```python
from build123d import *

# Parameters (mm, degrees)
SKETCH_1_R        = 1
EXTRUDE_1_DEPTH   = 1
SKETCH_1_2_R      = 1
EXTRUDE_1_2_DEPTH = 8
SKETCH_1_3_R      = 1
EXTRUDE_2_DEPTH   = 10
SCALE_4_SCALE     = 1.5


with BuildPart() as part:
    # 草图1 → Extrude 1 (new body)
    with BuildSketch(Plane.XY):
        with BuildLine():
            Line((-23.446136356, -44.161959762), (-25.73775467, -42.866863479))
            Line((-25.73775467, -42.866863479), (-26.834295942, -39.938466016))
            ThreePointArc((-26.834295942, -39.938466016), (-28.201527977, -38.125336415), (-30.335428898, -37.348658075))
            Line((-30.335428898, -37.348658075), (-33.334907776, -37.164700371))
            Line((-33.334907776, -37.164700371), (-33.842709051, -34.202800331))
            ThreePointArc((-33.842709051, -34.202800331), (-34.84597704, -32.165592505), (-36.7965457, -31.002818113))
            Line((-36.7965457, -31.002818113), (-39.708425324, -30.260072511))
            Line((-39.708425324, -30.260072511), (-39.652227319, -27.255483394))
            ThreePointArc((-39.652227319, -27.255483394), (-40.255989993, -25.066366444), (-41.954126526, -23.558687864))
            Line((-41.954126526, -23.558687864), (-44.675252109, -22.283466496))
            Line((-44.675252109, -22.283466496), (-44.057045667, -19.342627369))
            ThreePointArc((-44.057045667, -19.342627369), (-44.239914432, -17.079151855), (-45.625461503, -15.279979352))
            Line((-45.625461503, -15.279979352), (-48.059435816, -13.517457571))
            Line((-48.059435816, -13.517457571), (-46.901121207, -10.744549126))
            ThreePointArc((-46.901121207, -10.744549126), (-46.656617846, -8.486899797), (-47.680491761, -6.459969953))
            Line((-47.680491761, -6.459969953), (-49.741090048, -4.272585973))
            Line((-49.741090048, -4.272585973), (-48.083701146, -1.765839874))
            ThreePointArc((-48.083701146, -1.765839874), (-47.420487313, 0.406004917), (-48.046416828, 2.588887101))
            Line((-48.046416828, 2.588887101), (-49.660641368, 5.123644113))
            Line((-49.660641368, 5.123644113), (-47.562892001, 7.275425136))
            ThreePointArc((-47.562892001, 7.275425136), (-46.504462376, 9.284526705), (-46.710273625, 11.546031539))
            Line((-46.710273625, 11.546031539), (-47.82093971, 14.338366552))
            Line((-47.82093971, 14.338366552), (-45.357143694, 16.058954583))
            ThreePointArc((-45.357143694, 16.058954583), (-43.940993675, 17.834139505), (-43.719395692, 20.094152054))
            Line((-43.719395692, 20.094152054), (-44.287157421, 23.045145208))
            Line((-44.287157421, 23.045145208), (-41.54459596, 24.273587558))
            ThreePointArc((-41.54459596, 24.273587558), (-39.820893366, 25.751969023), (-39.17973637, 27.930427214))
            Line((-39.17973637, 27.930427214), (-39.184480502, 30.935538106))
            Line((-39.184480502, 30.935538106), (-36.260310201, 31.628316593))
            ThreePointArc((-36.260310201, 31.628316593), (-34.290118058, 32.757522199), (-33.252115355, 34.777253066))
            Line((-33.252115355, 34.777253066), (-32.693673826, 37.730024144))
            Line((-32.693673826, 37.730024144), (-29.691484877, 37.862596744))
            ThreePointArc((-29.691484877, 37.862596744), (-27.544598222, 38.602623821), (-26.146521576, 40.39207739))
            Line((-26.146521576, 40.39207739), (-25, 43.301270189))
            ThreePointArc((-25, 43.301270189), (-24.226890609, 43.73851588), (-23.446136356, 44.161959762))
            ThreePointArc((-23.446136356, 44.161959762), (-21.212806241, 47.755648425), (-21.906244367, 51.929556087))
            ThreePointArc((-21.906244367, 51.929556087), (-24.232021318, 53.76021953), (-27.179564099, 53.490852446))
            ThreePointArc((-27.179564099, 53.490852446), (-59.999999835, 0.004450967), (-27.1875, -53.486819346))
            Line((-27.1875, -53.486819346), (-27.179564099, -53.490852446))
            ThreePointArc((-27.179564099, -53.490852446), (-24.232021318, -53.76021953), (-21.906244367, -51.929556087))
            ThreePointArc((-21.906244367, -51.929556087), (-21.212806241, -47.755648425), (-23.446136356, -44.161959762))
        make_face()
        with Locations((-31.620079453, -45.001895242)):
            Circle(SKETCH_1_R, mode=Mode.SUBTRACT)
        with Locations((-55, 0)):
            Circle(SKETCH_1_R, mode=Mode.SUBTRACT)
        with Locations((-28.000624989, 47.338831842)):
            Circle(SKETCH_1_R, mode=Mode.SUBTRACT)
    extrude(amount=EXTRUDE_1_DEPTH)

    # 草图1<2> → Extrude 1 2 (add)
    with BuildSketch(Plane.XY):
        with BuildLine():
            Line((-23.446136356, -44.161959762), (-25.73775467, -42.866863479))
            Line((-25.73775467, -42.866863479), (-26.834295942, -39.938466016))
            ThreePointArc((-26.834295942, -39.938466016), (-28.201527977, -38.125336415), (-30.335428898, -37.348658075))
            Line((-30.335428898, -37.348658075), (-33.334907776, -37.164700371))
            Line((-33.334907776, -37.164700371), (-33.842709051, -34.202800331))
            ThreePointArc((-33.842709051, -34.202800331), (-34.84597704, -32.165592505), (-36.7965457, -31.002818113))
            Line((-36.7965457, -31.002818113), (-39.708425324, -30.260072511))
            Line((-39.708425324, -30.260072511), (-39.652227319, -27.255483394))
            ThreePointArc((-39.652227319, -27.255483394), (-40.255989993, -25.066366444), (-41.954126526, -23.558687864))
            Line((-41.954126526, -23.558687864), (-44.675252109, -22.283466496))
            Line((-44.675252109, -22.283466496), (-44.057045667, -19.342627369))
            ThreePointArc((-44.057045667, -19.342627369), (-44.239914432, -17.079151855), (-45.625461503, -15.279979352))
            Line((-45.625461503, -15.279979352), (-48.059435816, -13.517457571))
            Line((-48.059435816, -13.517457571), (-46.901121207, -10.744549126))
            ThreePointArc((-46.901121207, -10.744549126), (-46.656617846, -8.486899797), (-47.680491761, -6.459969953))
            Line((-47.680491761, -6.459969953), (-49.741090048, -4.272585973))
            Line((-49.741090048, -4.272585973), (-48.083701146, -1.765839874))
            ThreePointArc((-48.083701146, -1.765839874), (-47.420487313, 0.406004917), (-48.046416828, 2.588887101))
            Line((-48.046416828, 2.588887101), (-49.660641368, 5.123644113))
            Line((-49.660641368, 5.123644113), (-47.562892001, 7.275425136))
            ThreePointArc((-47.562892001, 7.275425136), (-46.504462376, 9.284526705), (-46.710273625, 11.546031539))
            Line((-46.710273625, 11.546031539), (-47.82093971, 14.338366552))
            Line((-47.82093971, 14.338366552), (-45.357143694, 16.058954583))
            ThreePointArc((-45.357143694, 16.058954583), (-43.940993675, 17.834139505), (-43.719395692, 20.094152054))
            Line((-43.719395692, 20.094152054), (-44.287157421, 23.045145208))
            Line((-44.287157421, 23.045145208), (-41.54459596, 24.273587558))
            ThreePointArc((-41.54459596, 24.273587558), (-39.820893366, 25.751969023), (-39.17973637, 27.930427214))
            Line((-39.17973637, 27.930427214), (-39.184480502, 30.935538106))
            Line((-39.184480502, 30.935538106), (-36.260310201, 31.628316593))
            ThreePointArc((-36.260310201, 31.628316593), (-34.290118058, 32.757522199), (-33.252115355, 34.777253066))
            Line((-33.252115355, 34.777253066), (-32.693673826, 37.730024144))
            Line((-32.693673826, 37.730024144), (-29.691484877, 37.862596744))
            ThreePointArc((-29.691484877, 37.862596744), (-27.544598222, 38.602623821), (-26.146521576, 40.39207739))
            Line((-26.146521576, 40.39207739), (-25, 43.301270189))
            ThreePointArc((-25, 43.301270189), (-24.226890609, 43.73851588), (-23.446136356, 44.161959762))
            ThreePointArc((-23.446136356, 44.161959762), (-21.212806241, 47.755648425), (-21.906244367, 51.929556087))
            ThreePointArc((-21.906244367, 51.929556087), (-24.232021318, 53.76021953), (-27.179564099, 53.490852446))
            ThreePointArc((-27.179564099, 53.490852446), (-59.999999835, 0.004450967), (-27.1875, -53.486819346))
            Line((-27.1875, -53.486819346), (-27.179564099, -53.490852446))
            ThreePointArc((-27.179564099, -53.490852446), (-24.232021318, -53.76021953), (-21.906244367, -51.929556087))
            ThreePointArc((-21.906244367, -51.929556087), (-21.212806241, -47.755648425), (-23.446136356, -44.161959762))
        make_face()
        with Locations((-31.620079453, -45.001895242)):
            Circle(SKETCH_1_2_R, mode=Mode.SUBTRACT)
        with Locations((-55, 0)):
            Circle(SKETCH_1_2_R, mode=Mode.SUBTRACT)
        with Locations((-28.000624989, 47.338831842)):
            Circle(SKETCH_1_2_R, mode=Mode.SUBTRACT)
    extrude(amount=EXTRUDE_1_2_DEPTH)

    # 草图1<3> → 凸台-拉伸2 (add)
    with BuildSketch(Plane.XY):
        with BuildLine():
            Line((-23.446136356, -44.161959762), (-25.73775467, -42.866863479))
            Line((-25.73775467, -42.866863479), (-26.834295942, -39.938466016))
            ThreePointArc((-26.834295942, -39.938466016), (-28.201527977, -38.125336415), (-30.335428898, -37.348658075))
            Line((-30.335428898, -37.348658075), (-33.334907776, -37.164700371))
            Line((-33.334907776, -37.164700371), (-33.842709051, -34.202800331))
            ThreePointArc((-33.842709051, -34.202800331), (-34.84597704, -32.165592505), (-36.7965457, -31.002818113))
            Line((-36.7965457, -31.002818113), (-39.708425324, -30.260072511))
            Line((-39.708425324, -30.260072511), (-39.652227319, -27.255483394))
            ThreePointArc((-39.652227319, -27.255483394), (-40.255989993, -25.066366444), (-41.954126526, -23.558687864))
            Line((-41.954126526, -23.558687864), (-44.675252109, -22.283466496))
            Line((-44.675252109, -22.283466496), (-44.057045667, -19.342627369))
            ThreePointArc((-44.057045667, -19.342627369), (-44.239914432, -17.079151855), (-45.625461503, -15.279979352))
            Line((-45.625461503, -15.279979352), (-48.059435816, -13.517457571))
            Line((-48.059435816, -13.517457571), (-46.901121207, -10.744549126))
            ThreePointArc((-46.901121207, -10.744549126), (-46.656617846, -8.486899797), (-47.680491761, -6.459969953))
            Line((-47.680491761, -6.459969953), (-49.741090048, -4.272585973))
            Line((-49.741090048, -4.272585973), (-48.083701146, -1.765839874))
            ThreePointArc((-48.083701146, -1.765839874), (-47.420487313, 0.406004917), (-48.046416828, 2.588887101))
            Line((-48.046416828, 2.588887101), (-49.660641368, 5.123644113))
            Line((-49.660641368, 5.123644113), (-47.562892001, 7.275425136))
            ThreePointArc((-47.562892001, 7.275425136), (-46.504462376, 9.284526705), (-46.710273625, 11.546031539))
            Line((-46.710273625, 11.546031539), (-47.82093971, 14.338366552))
            Line((-47.82093971, 14.338366552), (-45.357143694, 16.058954583))
            ThreePointArc((-45.357143694, 16.058954583), (-43.940993675, 17.834139505), (-43.719395692, 20.094152054))
            Line((-43.719395692, 20.094152054), (-44.287157421, 23.045145208))
            Line((-44.287157421, 23.045145208), (-41.54459596, 24.273587558))
            ThreePointArc((-41.54459596, 24.273587558), (-39.820893366, 25.751969023), (-39.17973637, 27.930427214))
            Line((-39.17973637, 27.930427214), (-39.184480502, 30.935538106))
            Line((-39.184480502, 30.935538106), (-36.260310201, 31.628316593))
            ThreePointArc((-36.260310201, 31.628316593), (-34.290118058, 32.757522199), (-33.252115355, 34.777253066))
            Line((-33.252115355, 34.777253066), (-32.693673826, 37.730024144))
            Line((-32.693673826, 37.730024144), (-29.691484877, 37.862596744))
            ThreePointArc((-29.691484877, 37.862596744), (-27.544598222, 38.602623821), (-26.146521576, 40.39207739))
            Line((-26.146521576, 40.39207739), (-25, 43.301270189))
            ThreePointArc((-25, 43.301270189), (-24.226890609, 43.73851588), (-23.446136356, 44.161959762))
            ThreePointArc((-23.446136356, 44.161959762), (-21.212806241, 47.755648425), (-21.906244367, 51.929556087))
            ThreePointArc((-21.906244367, 51.929556087), (-24.232021318, 53.76021953), (-27.179564099, 53.490852446))
            ThreePointArc((-27.179564099, 53.490852446), (-59.999999835, 0.004450967), (-27.1875, -53.486819346))
            Line((-27.1875, -53.486819346), (-27.179564099, -53.490852446))
            ThreePointArc((-27.179564099, -53.490852446), (-24.232021318, -53.76021953), (-21.906244367, -51.929556087))
            ThreePointArc((-21.906244367, -51.929556087), (-21.212806241, -47.755648425), (-23.446136356, -44.161959762))
        make_face()
        with Locations((-31.620079453, -45.001895242)):
            Circle(SKETCH_1_3_R, mode=Mode.SUBTRACT)
        with Locations((-55, 0)):
            Circle(SKETCH_1_3_R, mode=Mode.SUBTRACT)
        with Locations((-28.000624989, 47.338831842)):
            Circle(SKETCH_1_3_R, mode=Mode.SUBTRACT)
    extrude(amount=EXTRUDE_2_DEPTH)


with BuildPart() as part_1:
    # 缩放比例4: scaled about (-43.37819964, 0.034879878, 5)
    add(part.part.scale(SCALE_4_SCALE).moved(Location((21.68909982, -0.017439939, -2.5))))


solid = part_1.part
```
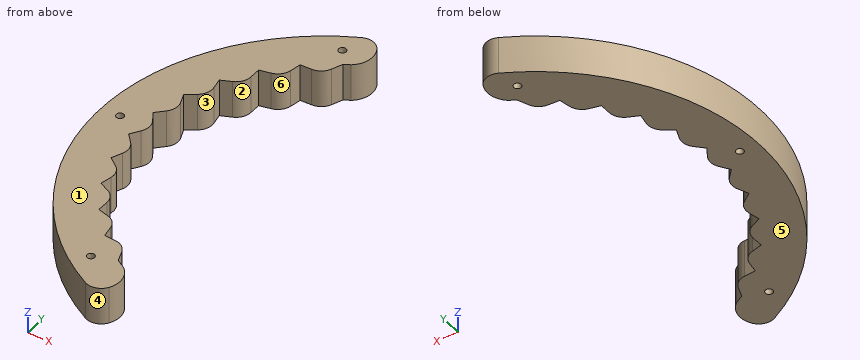
CAD build for the part. Positions are in the model's coordinates, mm. Face numbers are marked on the shaded views. A direction names the side the tool comes from. Coordinates: 2 decimals unless noted, no trailing zeros. Write each loop counter-clockwise with the first axis right and the second up, starting at its lowest first coordinate (ties: lowest second). Pieces come first, ordered by that corner, then holes.
(1) Cut at C-C, the plane y = -53. List the corners of the cut face in (x, z), and give its area (3 significant figures).
(2) Flat gauge pins, fed straight in: pin 1 (5 mm diameter, centred on x = -56, z = 3.5, fed in from +Y); pin 2 (8 mm diameter, centred on y = 26.5, z = 9, fed in from +X); pin 3 (2.5 mm diameter, centred on x = -20.31, y = 70.99, fed in from +Z); pin 4 (6 mm diameter, centred on x = -21, z = 9.5, fed in from -Y). Where does each tip first touch, or does it go through?
(3) Cut at A-A, the plane x = -35. List the corners of the cut face in (y, z).
(4) 3-axis set-ups, long thin cutter, end or side, ignore diameter. For the marked faces 1 and 2: which of +Z, -Z, +X, -X, +Y, -Y reach the whole face in a straight line?
(5) Cut at D-D, the plane y = 32.5. List the corners of the cut face in (x, z), and give its area (3 significant figures).
(6) Cut at B-B, the plane z = 2.25. Count the separate pieces of the cut face and the enclosed holes in it, and give its area (3 significant figures).
(7) Two-plate mould, pull along Y, no slides. Class the marked faces 3, 4, 5 and 6: +Y half, -Y half, draft (parallel to the pull), parting line (faces both ways), or undercut.
(8) Drill centre lines: probe 1 along X at (y, z) = (0, 1.5); probe 2 along Y at (x, z) = (-25, 5.25); probe 3 along X at (y, z) = (-68, 7.25). Where is each one in solid material? Low to high.
Geometry says:
1. outline: (-51.06, -2.5) - (-28.79, -2.5) - (-28.79, 12.5) - (-51.06, 12.5) - close
1. area: 334 mm2
2. pin 1: stops at y = 49.45
2. pin 2: stops at x = -43.78
2. pin 3: passes through
2. pin 4: stops at y = -80.68
3. outline: (-69.92, -2.5) - (-46.14, -2.5) - (-46.14, 12.5) - (-69.92, 12.5) - close; (46.88, -2.5) - (69.88, -2.5) - (69.88, 12.5) - (46.88, 12.5) - close
4. face 1: +Z, +X, -X, +Y, -Y
4. face 2: +Z, -Z, +X
5. outline: (-62.23, -2.5) - (-44.35, -2.5) - (-44.35, 12.5) - (-62.23, 12.5) - close
5. area: 268 mm2
6. separate pieces: 1
6. enclosed holes: 3
6. area: 3,210 mm2
7. face 3: undercut
7. face 4: -Y half
7. face 5: draft
7. face 6: undercut
8. probe 1: x = -68.31 to -62.31, -59.31 to -49.48
8. probe 2: y = -76.96 to -68.82, -66.22 to -55.97, 56.68 to 76.92
8. probe 3: x = -37.29 to -27.16, -24.32 to -11.76
